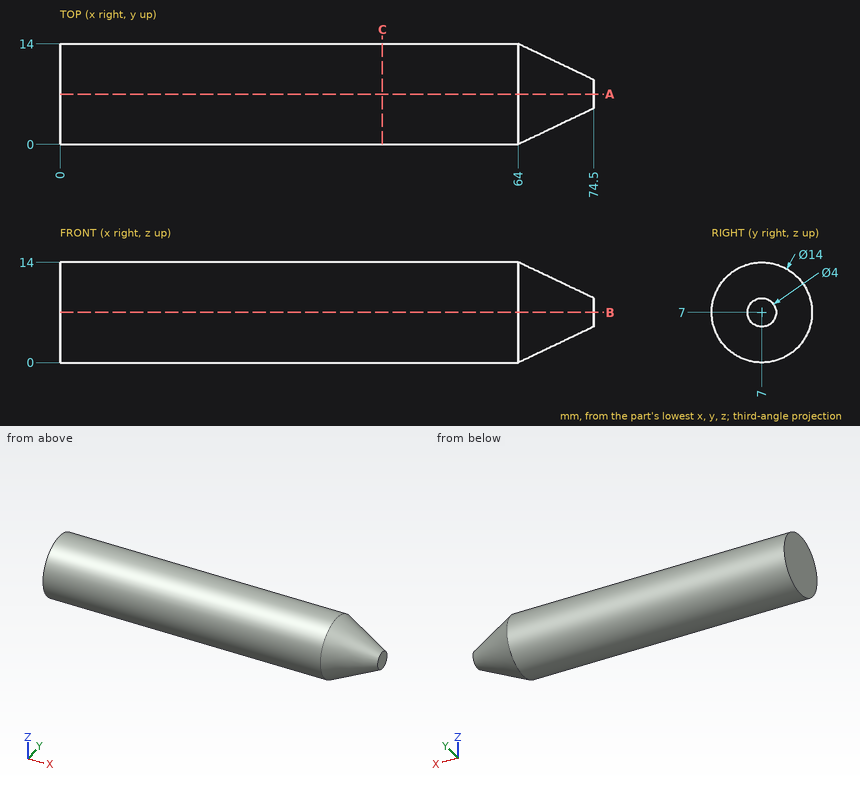
Study the drawing (mm; zero at the part's minimum x, y, z) and answer. Give positions to 0.01 mm unless a question says otherwise; leave off trailing zeros. Order: outer loops, then holes, each group sorted by start corner. A loop starts at its lowest first (then second) coordinate and runs counter-clockwise, first axis right, second up. Notation, with made-up numbers: M -35.75,66.5 L 8.25,66.5 A21 ccw 8.25,96.5 Z; hole C 21,-31.5 d6. An arc over 180 degrees is marked long. Put each result on its own line as item: value. Start each with the question number.
Item 1: The part is cut by section C-C, the plane x = 45. Determine the outline of the cut face in (y, z), and give its area (3 significant figures).
Item 2: Flat-ended cylindrical pins translate along their axes: P1, Ø4, axis at x = 18, y = 3, coming from the -Z side; P2, Ø1.5, axis at x = 55, z = 10.5, coming from the -Y side; P3, Ø2, axis at x = 57, y = 9, coming from the +Z side. Find the tip coordinate at first contact, or state that the pin passes through.
Item 3: Find the intervals of material crossed by line 1 along Z through (x, y) = (10, 6.75); line 2 along Y through (x, z) = (37, 11); line 3 along X through (y, z) = (6.5, 2.75), in increasing order.
Item 4: The part is cut by section A-A, the plane y = 7. Determine the outline of the cut face in (x, z).
Answer key:
1. outline: C 7,7 d14
1. area: 154 mm²
2. P1: stops at z = 0.29
2. P2: stops at y = 0.56
2. P3: stops at z = 13.93
3. line 1: z = 0 to 14
3. line 2: y = 1.26 to 12.74
3. line 3: x = 0 to 69.71
4. outline: M 0,0 L 64,0 L 74.5,5 L 74.5,9 L 64,14 L 0,14 Z
